For this review, take the finished solid that the model builds, in its own axes (mm). A direction names the side the tool comes from. Coordinates: 2 decimals unless noted, no trailing zeros. Write each loop counter-clockwise with the first axis right and the second up, starting at its lowest first coordinate (ties: lowest second). Pieces come first, ordered by that corner, then holes.
1) We need section D-D on z = -34.5. Write out the cut boundary in (x, y), then the cut area to 3 significant figures.
2) Mouldability with a two-part tool opening along X and no side actions: class faces 1 (the face through (-34.79, 5.476, 4.336)), 2 (the face through (50, 74, 1)), 3 (the face through (20, 49, 1)) as pulls with the +X half, pulls with the -X half, needs draft (parallel to the pull), parting line crosses it, or undercut.
3) We need section B-B on z = 0. Write out the cut boundary in (x, y).
4) We need section C-C on x = 32. Write out the cut boundary in (y, z), then the cut area to 3 significant figures.
5) Insertion check: P1, Ø1.5, axis at x = -16.5, z = -29, coming from the -Y side; P2, Ø1.5, axis at y = 160.5, z = -14, coming from the -X side. Each pin has a flat end and moves straight along its axis. Give the tip position at first contact, or say it passes through.
6) For faces 4 (the face through (7.509, 199.3, 23.846)), 5 (the face through (-35, 0, -1)), 6 (the face through (0, 100, -1)), list the 3-axis set-ups (+Z, -Z, +X, -X, +Y, -Y) from which the entire face can be reached by the end or side of a thin tool; tool diameter is ignored.
7) To check wall thickness, follow line 1 along Y through (x, z) = (43, 0); line 2 along X through (y, z) = (14.5, -44); line 3 along Z through (x, y) = (-29.5, 23.5). State the ranges of each line that lie inside material, in increasing order.
8) We need section A-A on y = 25. Write out the cut boundary in (x, z), then the cut area to 3 significant figures.
from build123d import *

# Parameters (mm, degrees)
SKETCH1_W             = 30
SKETCH1_H             = 120
BOSS_EXTRUDE1_DEPTH   = 100
BOSS_EXTRUDE1_2_DEPTH = 100
SKETCH2_R             = 20
CUT_EXTRUDE1_DEPTH    = 150
SKETCH3_W             = 100
SKETCH3_H             = 120
BOSS_EXTRUDE2_DEPTH   = 50
SKETCH4_R             = 25
BOSS_EXTRUDE3_DEPTH   = 100


with BuildPart() as part:
    # Sketch1 → Boss-Extrude1 (new body)
    with BuildSketch(Plane(origin=(0, 0, 0), x_dir=(1, 0, 0), z_dir=(0, 1, 0))):
        with Locations((-35, 0)):
            Rectangle(SKETCH1_W, SKETCH1_H)
    extrude(amount=BOSS_EXTRUDE1_DEPTH)


with BuildPart() as body_2:
    # Sketch1 → Boss-Extrude1 2 (new body)
    with BuildSketch(Plane(origin=(0, 0, 0), x_dir=(1, 0, 0), z_dir=(0, 1, 0))):
        with Locations((35, 0)):
            Rectangle(SKETCH1_W, SKETCH1_H)
    extrude(amount=BOSS_EXTRUDE1_2_DEPTH)


with BuildPart() as cut_extrude1_tool:
    # Sketch2 → Cut-Extrude1 (new body)
    with BuildSketch(Plane(origin=(50, 0, 0), x_dir=(0, 0, -1), z_dir=(1, 0, 0))):
        with Locations((0, 25)):
            Circle(SKETCH2_R)
    extrude(amount=-CUT_EXTRUDE1_DEPTH)


with BuildPart() as part_1:
    add(part.part)

    # Cut-Extrude1: cut by cut_extrude1_tool
    add(cut_extrude1_tool.part, mode=Mode.SUBTRACT)



with BuildPart() as body_2_1:
    add(body_2.part)

    # Cut-Extrude1: cut by cut_extrude1_tool
    add(cut_extrude1_tool.part, mode=Mode.SUBTRACT)


with BuildPart() as part_2:
    add(part_1.part)

    add(body_2_1.part)  # Boss-Extrude2 merges body 2
    # Sketch3 → Boss-Extrude2 (add)
    with BuildSketch(Plane(origin=(0, 100, 0), x_dir=(1, 0, 0), z_dir=(0, 1, 0))):
        Rectangle(SKETCH3_W, SKETCH3_H)
    extrude(amount=BOSS_EXTRUDE2_DEPTH)

    # Sketch4 → Boss-Extrude3 (add)
    with BuildSketch(Plane(origin=(0, 150, 0), x_dir=(1, 0, 0), z_dir=(0, 1, 0))):
        with Locations(Location((0, 0, 0), (0, 0, 270))):
            Circle(SKETCH4_R)
    extrude(amount=BOSS_EXTRUDE3_DEPTH)


solid = part_2.part
Result:
1. outline: (-50, 0) - (-20, 0) - (-20, 100) - (20, 100) - (20, 0) - (50, 0) - (50, 150) - (-50, 150) - close
1. area: 11,000 mm2
2. face 1: needs draft
2. face 2: pulls with the +X half
2. face 3: undercut
3. outline: (-50, 0) - (-20, 0) - (-20, 5) - (-50, 5) - close; (-50, 45) - (-20, 45) - (-20, 100) - (20, 100) - (20, 45) - (50, 45) - (50, 150) - (25, 150) - (25, 250) - (-25, 250) - (-25, 150) - (-50, 150) - close; (20, 0) - (50, 0) - (50, 5) - (20, 5) - close
4. outline: (0, -60) - (150, -60) - (150, 60) - (0, 60) - close; hole circle Ø40 at (25, 0)
4. area: 16,700 mm2
5. P1: stops at y = 100
5. P2: stops at x = -21.2
6. face 4: +Y
6. face 5: +Z, -Z, +X, -X, -Y
6. face 6: +Z, -Z, -Y
7. line 1: y = 0 to 5, 45 to 150
7. line 2: x = -50 to -20, 20 to 50
7. line 3: z = -60 to -19.94, 19.94 to 60
8. outline: (-50, -60) - (-20, -60) - (-20, -20) - (-50, -20) - close; (-50, 20) - (-20, 20) - (-20, 60) - (-50, 60) - close; (20, -60) - (50, -60) - (50, -20) - (20, -20) - close; (20, 20) - (50, 20) - (50, 60) - (20, 60) - close
8. area: 4,800 mm2
